Part model, mm, in its own coordinate system. A direction names the side the tool comes from. Coordinates: 2 decimals unless noted, no trailing zeros. Loops run counter-clockwise (first coordinate to the right, second up) from the corner with the lowest first, then second, coordinate; pieces in that order, holes last. Notation, with made-up numbers: M 13,75.5 L 56,75.5 A23 cw 56,101.5 Z; hole C -20.75,4 d8. An arc over 180 degrees is marked long. Answer as CSV lines item,"result". Start each with the question number.
Autodesk Inventor part; units mm, degrees
ref_plane "YZ Plane" through (0, 0, 0) normal (1, 0, 0) x (0, 1, 0)
ref_plane "XZ Plane" through (0, 0, 0) normal (0, 1, 0) x (-1, 0, 0)
ref_plane "XY Plane" through (0, 0, 0) normal (0, 0, 1) x (1, 0, 0)
sketch "Sketch9" plane through (0, 0, 0) normal (0, 1, 0) x (-1, 0, 0)
  line L0 (15, 15) -> (-15, 15)
  line L1 (-15, 15) -> (-15, -15)
  line L2 (-15, -15) -> (15, -15)
  line L3 (15, -15) -> (15, 15)
  line L4 (15, 15) -> (-15, -15) construction
  line L5 (-15, 15) -> (15, -15) construction
  line L6 (-13, 13) -> (13, 13)
  line L7 (13, 13) -> (13, -13)
  line L8 (13, -13) -> (-13, -13)
  line L9 (-13, -13) -> (-13, 13)
  point P0 (0, 0)
  dimension "d172" = 30
  dimension "d173" = 30
  dimension "d174" = 2
extrude "Extrusion3" add sketch "Sketch9" against normal blind 340
sketch "Sketch10" plane through (0, 0, 0) normal (1, 0, 0) x (0, 1, 0)
  line L0 (0, 15) -> (0, -15) construction
  line L1 (0, 15) -> (-340, 15) construction
  line L2 (-340, -15) -> (-340, 15) construction
  line L3 (0, -15) -> (-340, -15) construction
  line L4 (-68.5, 8.5) -> (-51.5, 8.5)
  line L5 (-51.5, 8.5) -> (-51.5, -8.5)
  line L6 (-51.5, -8.5) -> (-68.5, -8.5)
  line L7 (-68.5, -8.5) -> (-68.5, 8.5)
  line L8 (-68.5, 8.5) -> (-51.5, -8.5) construction
  line L9 (-51.5, 8.5) -> (-68.5, -8.5) construction
  line L10 (0, 0) -> (30, 0)
  circle A0 centre (-60, 0) radius 8.5
  dimension "d177" = 17
  dimension "d178" = 17
  dimension "d181" = 30
  dimension "d182" = 90
extrude "Extrusion4" cut sketch "Sketch10" along normal through all contours A0
pattern_linear "Rectangular Pattern4" count 4 spacing 85 along (0, -1, 0) of "Extrusion4"
properties part number "SLM 1661 FDS 1000 way tube 1" material "Stainless Steel"
Q1. Tool access for faces 5 (the face through (13.99, -68.49, -0.37)), 6 (the face through (-13, -168, 0)), 7 (the face through (15, -168, 0)): list every direction of +Z, -Z, +X, -X, +Y, -Y with a clear straight run to the whole face (end or side of a thin tool).
Q2. Wall check: L1, parallel to Y at x = 14.3, z = 0; L2, parallel to Z at x = 11.5, y = -233. Give the ranges that are in metal, low to high.
Q3. Slice it at C-C, the plane z = 0. Write the cut outline in (x, y).
Q4. Slice it at B-B, the plane y = -301.5. Write the cut outline in (x, z).
Q5. Slice it at D-D, the plane y = -60. Write the cut outline in (x, z), and give its area (3 significant figures).
Q6. Slice it at A-A, the plane x = -9. Write the cut outline in (y, z), and give its area (3 significant figures).
Q7. Two-plate mould, pull along X, no slides. Class faces 1 (the face through (13.99, -238.49, -0.37)), 2 (the face through (0, -168, 13)), 3 (the face through (0, -168, -13)), 4 (the face through (-15, -168, 0)): +X half, -X half, draft (parallel to the pull), parting line (faces both ways), or undercut.
Q8. Flat gauge pin, fed straight in: P1, Ø10, axis at y = -145, z = 0, coming from the +X side. Where does the tip first touch, or does it go through?
Solved:
1,face 5,"+X"
1,face 6,"+Y, -Y"
1,face 7,"+Z, -Z, +X, +Y, -Y"
2,L1,"y = -340 to -323.5, -306.5 to -238.5, -221.5 to -153.5, -136.5 to -68.5, -51.5 to 0"
2,L2,"z = -15 to -13, 13 to 15"
3,outline,"M -15,-340 L -13,-340 L -13,0 L -15,0 Z; M 13,-340 L 15,-340 L 15,-323.5 L 13,-323.5 Z; M 13,-306.5 L 15,-306.5 L 15,-238.5 L 13,-238.5 Z; M 13,-221.5 L 15,-221.5 L 15,-153.5 L 13,-153.5 Z; M 13,-136.5 L 15,-136.5 L 15,-68.5 L 13,-68.5 Z; M 13,-51.5 L 15,-51.5 L 15,0 L 13,0 Z"
4,outline,"M -15,-15 L 15,-15 L 15,15 L -15,15 Z; hole M -13,-13 L 13,-13 L 13,13 L -13,13 Z"
5,outline,"M -15,-15 L 15,-15 L 15,-8.5 L 13,-8.5 L 13,-13 L -13,-13 L -13,13 L 13,13 L 13,8.5 L 15,8.5 L 15,15 L -15,15 Z"
5,area,"190 mm2"
6,outline,"M -340,-15 L 0,-15 L 0,-13 L -340,-13 Z; M -340,13 L 0,13 L 0,15 L -340,15 Z"
6,area,"1,360 mm2"
7,face 1,"draft"
7,face 2,"undercut"
7,face 3,"undercut"
7,face 4,"-X half"
8,P1,"stops at x = -13"
